Check sheet for the modelled part. Datum: model origin and axes. Units: mm. A direction names the side the tool comes from. Coordinates: 2 decimals unless noted, no trailing zeros. Order: outer loops, then holes, each group sorted by start corner. A loop starts at its lowest first (then second) coordinate and runs counter-clockwise, first axis right, second up. Notation, with made-up numbers: M -6,-10 L 10,-10 A12 cw 10,5 Z; hole C -5,-10.5 d8. An arc over 180 degrees is marked long. Answer in a Markdown table with one row per item. Add a question column.
from build123d import *

# Parameters (mm, degrees)
ESQUISSE1_W             = 156
ESQUISSE1_H             = 84
BOSS_EXTRU_1_DEPTH      = 59
ESQUISSE2_W             = 78
ESQUISSE2_H             = 16
ESQUISSE2_W_2           = 7
ESQUISSE2_H_2           = 35
ESQUISSE2_W_3           = 4.2
ESQUISSE2_H_3           = 2.5
ENL_V_MAT_EXTRU_1_DEPTH = 177.572550515
ENL_V_MAT_EXTRU_3_DEPTH = 141.546285889
ESQUISSE4_W             = 52
ESQUISSE4_H             = 20
ENL_V_MAT_EXTRU_4_DEPTH = 59
BOSS_EXTRU_2_DEPTH      = 34
BOSS_EXTRU_3_DEPTH      = 34


with BuildPart() as part:
    # Esquisse1 → Boss.-Extru.1 (new body)
    with BuildSketch(Plane(origin=(0, 0, 0), x_dir=(1, 0, 0), z_dir=(0, 1, 0))):
        with Locations((23.701811573, 15.972972973)):
            Rectangle(ESQUISSE1_W, ESQUISSE1_H)
    extrude(amount=BOSS_EXTRU_1_DEPTH)

    # Esquisse2 → Enlèv. mat.-Extru.1 (cut, through all)
    with BuildSketch(Plane(origin=(101.701811573, 0, 0), x_dir=(0, 0, -1), z_dir=(1, 0, 0))):
        Polygon((15.972972973, 24), (47.972972973, 24), (47.972972973, 56), (-16.027027027, 56), (-16.027027027, 24), align=None)
        with Locations((15.972972973, 13)):
            Rectangle(ESQUISSE2_W, ESQUISSE2_H)
        with Locations((-22.527027027, 41.5)):
            Rectangle(ESQUISSE2_W_2, ESQUISSE2_H_2)
        Polygon((54.972972973, 24), (57.972972973, 24), (57.972972973, 59), (50.972972973, 59), (50.972972973, 24), align=None)
        with Locations((24.072972973, 1.25)):
            Rectangle(ESQUISSE2_W_3, ESQUISSE2_H_3)
    extrude(amount=-ENL_V_MAT_EXTRU_1_DEPTH, mode=Mode.SUBTRACT)

    # Esquisse3 → Enlèv. mat.-Extru.3 (cut, through all)
    with BuildSketch(Plane.XY.offset(19.027027027)):
        with BuildLine():
            Line((101.701811573, 59), (40.701811573, 59))
            add(Edge.make_bspline(
                [(40.701811573, 59), (63.23269898, 27.796698054), (101.701811573, 24)],
                knots=[0, 0, 0, 1, 1, 1], degree=2))
            Line((101.701811573, 24), (101.701811573, 59))
        make_face()
    extrude(amount=-ENL_V_MAT_EXTRU_3_DEPTH, mode=Mode.SUBTRACT)

    # Esquisse4 → Enlèv. mat.-Extru.4 (cut)
    with BuildSketch(Plane.XY.offset(19.027027027)):
        with Locations((-25.298188427, 34)):
            Rectangle(ESQUISSE4_W, ESQUISSE4_H)
    extrude(amount=-ENL_V_MAT_EXTRU_4_DEPTH, mode=Mode.SUBTRACT)

    # Esquisse5 → Boss.-Extru.2 (add)
    with BuildSketch(Plane(origin=(0, 0, -57.972972973), x_dir=(-1, 0, 0), z_dir=(0, 0, -1))):
        Polygon((-101.701811573, 2.5), (-40.701811573, 2.75), (-40.701811573, 5.5), (-101.701811573, 5.5), align=None)
        Polygon((-40.701811573, 2.75), (-6.701811573, 2.660526316), (-6.701811573, 5.5), (-40.701811573, 5.5), align=None)
    extrude(amount=BOSS_EXTRU_2_DEPTH)

    # Esquisse6 → Boss.-Extru.3 (add)
    with BuildSketch(Plane.XY.offset(26.027027027)):
        Polygon((-54.298188427, 2.5), (-54.298188427, 0), (101.701811573, 0), (101.701811573, 2.5), (6.701811573, 2.5), (6.701811573, 5.5), (101.701811573, 5.5), (101.701811573, 24), (-54.298188427, 24), (-54.298188427, 5.5), align=None)
    extrude(amount=BOSS_EXTRU_3_DEPTH)


solid = part.part
1. Section check A-A on y = 18.5. Enter the section's corners in (x, z).
2. Set-up check for faces 4 (the flat face through (25, 24, -54)), 5 (the flat face through (25, 41, 19.027)), 6 (the flat face through (25, 2.5, -24)), 7 (the flat face through (7, 40, -47.973)), 8 (the flat face through (-54.298, 23, 18)): record each of +Z, -Z, +X, -X, +Y, -Y from which the full face is reachable in a straight line by a thin tool's end or side.
3. Section check C-C on x = 3.5. Enter the section's corners in (y, z).
4. Section check B-B on x = -31.5. Enter the section's corners in (y, z), then the cut area to 3 significant figures.
5. Release check for a two-part mould opening along Y. For faces 1 (the flat face through (25, 13, -54.973)), 2 (the flat face through (23, 12, -57.973)), 3 (the flat face through (23, 0, 18)) record: released by +Y, released by -Y, zero draft, split by the parting line, or undercut.
6. Scan lines: line 1 (Y direction, x = 25, z = -29); line 2 (Y direction, x = 90.5, z = -43); line 3 (Z direction, x = 12, y = 42.5). Record each from-to range of solid material in increasing order.
7. Go/stop test with flat-tipped pins: pin 1 Ø0.9 at (y, z) = (4, -82.5) entering from -X; pin 2 Ø3.5 at (y, z) = (4, 35.5) entering from +X; pin 3 Ø8 at (y, z) = (53, 2.5) entering from +X; pin 4 Ø4 at (x, z) = (54.5, 39) entering from +Y. Record where each tip stops, or that it passes through.
8. Section check D-D on z = -20. State how many separate pieces and enclosed holes the cut face has, then the cut area to 3 significant figures.
Result sheet:
| question | item | result |
|---|---|---|
| 1 | outline | M -54.3,-57.97 L 101.7,-57.97 L 101.7,-54.97 L -54.3,-54.97 Z; M -54.3,23.03 L 101.7,23.03 L 101.7,60.03 L -54.3,60.03 Z |
| 2 | face 4 | -Z, +X, -X, +Y |
| 2 | face 5 | +Z, +X, -X, +Y |
| 2 | face 6 | +X, -X, -Y |
| 2 | face 7 | +X, -X |
| 2 | face 8 | +Z, -Z, -X, +Y, -Y |
| 3 | outline | M 0,-57.97 L 24,-57.97 L 24,-50.97 L 59,-50.97 L 59,19.03 L 24,19.03 L 24,60.03 L 0,60.03 L 0,-21.97 L 2.5,-21.97 L 2.5,-26.17 L 0,-26.17 Z; hole M 5,-54.97 L 21,-54.97 L 21,23.03 L 5,23.03 Z; hole M 24,-47.97 L 56,-47.97 L 56,16.03 L 24,16.03 Z |
| 4 | outline | M 0,-57.97 L 24,-57.97 L 24,-50.97 L 59,-50.97 L 59,19.03 L 44,19.03 L 44,16.03 L 56,16.03 L 56,-47.97 L 24,-47.97 L 24,60.03 L 0,60.03 L 0,-21.97 L 2.5,-21.97 L 2.5,-26.17 L 0,-26.17 Z; hole M 5,-54.97 L 21,-54.97 L 21,23.03 L 5,23.03 Z |
| 4 | area | 1,920 mm^2 |
| 5 | face 1 | undercut |
| 5 | face 2 | zero draft |
| 5 | face 3 | released by -Y |
| 6 | line 1 | 0 to 5, 21 to 24, 56 to 59 |
| 6 | line 2 | 0 to 5, 21 to 24 |
| 6 | line 3 | -50.97 to -47.97, 16.03 to 19.03 |
| 7 | pin 1 | x = 6.7 |
| 7 | pin 2 | x = 101.7 |
| 7 | pin 3 | x = 42.95 |
| 7 | pin 4 | y = 24 |
| 8 | separate pieces | 3 |
| 8 | enclosed holes | 0 |
| 8 | area | 1,540 mm^2 |
